Can you work these out from the model? Positions are in its coordinate system, mm. Face numbers are marked on the shaded views. Round coordinates to 2 decimals unless told otherwise and drop trailing zeros. Loops run counter-clockwise (first coordinate to the right, second up) from the corner with the lowest first, then second, coordinate; pieces in that order, holes last.
(1) If I drill on line 1 along Y through (x, z) = (4.75, 2.5); line 2 along Z through (x, y) = (8.5, 6); line 3 along Y through (x, z) = (2.75, 1.5), over which ranges is the centre line in solid material (lowest first)?
(2) I want a section at A-A on z = 5.5. Write out the boundary of the cut face in (x, y), plus the area to 3 significant figures.
(3) Will these pins go through, and if not, where does the flat tip stop? pin 1 Ø6 at (x, y) = (8, 34.5) entering from +Z; pin 2 Ø2 at (x, z) = (7.5, 3) entering from +Y.
(4) I want a section at B-B on x = 2.25. Write out the boundary of the cut face in (y, z).
(5) Thinking about a two-plate mould opening in Y: for the marked faces 1 and 2, which applies, released by +Y, released by -Y, zero draft, split by the parting line, or undercut?
from build123d import *

# Parameters (mm, degrees)
F1_DEPTH    = 6.604
F2_T2_ANGLE = 37.6266885083
F2_T4_ANGLE = 37.6266885083
F3_T1_DEPTH = 39.1771149622
F4_T2_ANGLE = 30.7081908039
F4_T4_ANGLE = 30.7081908039


# Not quite as in the source:
# - a fillet or chamfer that OpenCascade refuses, or shapes differently, is made with other operations: its cross-section is extruded or revolved along the edge and cut away or added
# - ends of sketch curves that miss each other by under 0.0002 mm in the source are joined


with BuildPart() as f1:
    # F0 (on Top) → F1 (new body)
    with BuildSketch(Plane.XY):
        with BuildLine():
            Line((0, 76.2824639678), (0, 0))
            Line((0, 0), (13.1280263886, 0))
            ThreePointArc((13.1280263886, 0), (9.4882529844, 31.2224067748), (13.1280263886, 62.4448174897))
            Line((13.1280263886, 62.4448174897), (0, 76.2824639678))
        make_face()
        with BuildLine():
            Line((13.1280263886, 0), (0, 0))
            Line((0, 0), (0, -48.9660091698))
            ThreePointArc((0, -48.9660091698), (4.8963223511, -56.1371050306), (13.1280263886, -58.900732547))
            ThreePointArc((13.1280263886, -58.900732547), (9.9051564545, -29.4503682436), (13.1280263886, 0))
        make_face()
    extrude(amount=F1_DEPTH)

    # F2: chamfer of 5.08 on 2 edges, made by hand

    # F2_s1 → F2_t2 (revolve, cut)
    with BuildSketch(Plane(origin=(5.5719325615, -16.3549575283, 0), x_dir=(0, 0, 1), z_dir=(0.3224861622, -0.9465741784, 0))):
        Polygon((1.524, -11.7983946988), (6.604, -6.7183946988), (6.604, -11.7983946988), align=None)
    revolve(axis=Axis((145.2229057415, 31.2224087449, 6.604), (0, 0, -1)), revolution_arc=F2_T2_ANGLE, mode=Mode.SUBTRACT)

    # F2_s3 → F2_t4 (revolve, cut)
    with BuildSketch(Plane(origin=(5.5719325615, -16.3549575283, 0), x_dir=(0, 0, 1), z_dir=(0.3224861622, -0.9465741784, 0))):
        Polygon((5.08, -11.7983946988), (0, -6.7183946988), (0, -11.7983946988), align=None)
    revolve(axis=Axis((145.2229057415, 31.2224087449, 0), (0, 0, -1)), revolution_arc=F2_T4_ANGLE, mode=Mode.SUBTRACT)

    # F3: chamfer of 5.08 on 2 edges, made by hand

    # F3_s2 → F3_t1 (cut)
    with BuildSketch(Plane(origin=(-20.115918924, 21.2032613595, 0), x_dir=(0, 0, 1), z_dir=(-0.6882605094, 0.725463625, 0))):
        Polygon((5.08, 52.5022075061), (0, 47.4222075061), (0, 52.5022075061), align=None)
        Polygon((1.524, 52.5022075061), (6.604, 47.4222075061), (6.604, 52.5022075061), align=None)
    extrude(amount=F3_T1_DEPTH, mode=Mode.SUBTRACT)

    # F4: fillet of radius 5.08 on 2 edges, made by hand

    # F4_s1 → F4_t2 (revolve, cut)
    with BuildSketch(Plane(origin=(22.2878822439, -69.2757873609, 0), x_dir=(0, 0, 1), z_dir=(0.3062665426, -0.9519457994, 0))):
        with BuildLine():
            ThreePointArc((6.604, 11.2139897709), (5.1161024484, 7.6218873224), (1.524, 6.1339897709))
            Line((1.524, 6.1339897709), (6.604, 6.1339897709))
            Line((6.604, 6.1339897709), (6.604, 11.2139897709))
        make_face()
    revolve(axis=Axis((146.0743134808, -29.4503662735, 6.604), (0, 0, -1)), revolution_arc=F4_T2_ANGLE, mode=Mode.SUBTRACT)

    # F4_s3 → F4_t4 (revolve, cut)
    with BuildSketch(Plane(origin=(22.2878822439, -69.2757873609, 0), x_dir=(0, 0, 1), z_dir=(0.3062665426, -0.9519457994, 0))):
        with BuildLine():
            ThreePointArc((0, 11.2139897709), (1.4878975516, 7.6218873224), (5.08, 6.1339897709))
            Line((5.08, 6.1339897709), (0, 6.1339897709))
            Line((0, 6.1339897709), (0, 11.2139897709))
        make_face()
    revolve(axis=Axis((146.0743134808, -29.4503662735, 0), (0, 0, -1)), revolution_arc=F4_T4_ANGLE, mode=Mode.SUBTRACT)


solid = f1.part
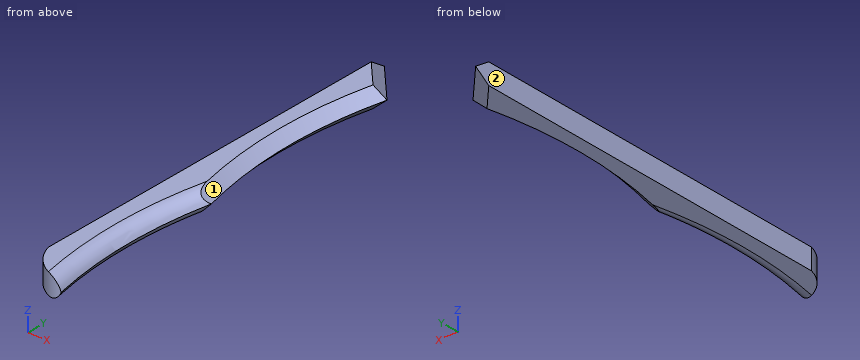
Filled sheet:
1. line 1: y = -56.02 to 67.53
1. line 2: z = 1.78 to 4.82
1. line 3: y = -54.11 to 68.18
2. outline: (0, -48.97) arc R13.64 ccw to (11.13, -58.75) arc R138.09 cw to (10.22, -4.73) arc R139.71 cw to (8.78, 61.25) - (0, 70.51) - close
2. area: 941 mm2
3. pin 1: stops at z = 6.05
3. pin 2: stops at y = 66.8
4. outline: (-53.49, 0) - (66.53, 0) - (71.33, 3.3) - (66.53, 6.6) - (-53.49, 6.6) - close
5. face 1: undercut
5. face 2: zero draft
